```python
from build123d import *

# Parameters (mm, degrees)
SKETCH1_W           = 78.74
SKETCH1_H           = 127
SKETCH1_W_2         = 38.1
SKETCH1_H_2         = 44.45
BOSS_EXTRUDE1_DEPTH = 2.54
BOSS_EXTRUDE2_DEPTH = 44.45
CUT_EXTRUDE1_REACH  = 129
SKETCH3_W           = 9.5
SKETCH3_H           = 11.5
SKETCH3_W_2         = 13
CUT_EXTRUDE2_REACH  = 103.6
CUT_EXTRUDE3_REACH  = 121.38
SKETCH6_R           = 3
SKETCH29_R          = 9.144
SKETCH29_R_2        = 6.604
CUT_EXTRUDE8_DEPTH  = 2.54


with BuildPart() as part:
    # Sketch1 → Boss-Extrude1 (new body)
    with BuildSketch(Plane(origin=(0, 0, 0), x_dir=(1, 0, 0), z_dir=(0, 1, 0))):
        with Locations((39.37, 63.5)):
            Rectangle(SKETCH1_W, SKETCH1_H)
        with Locations((97.79, 104.775)):
            Rectangle(SKETCH1_W_2, SKETCH1_H_2)
        Polygon((116.84, 127), (116.84, 82.55), (116.84, 0), (177.8, 0), (177.8, 127), align=None)
    extrude(amount=BOSS_EXTRUDE1_DEPTH)

    # Sketch2 → Boss-Extrude2 (add)
    with BuildSketch(Plane(origin=(0, 2.54, 0), x_dir=(1, 0, 0), z_dir=(0, 1, 0))):
        Polygon((0, 127), (0, 0), (78.74, 0), (78.74, 82.55), (116.84, 82.55), (116.84, 0), (177.8, 0), (177.8, 127), align=None)
        Polygon((119.38, 2.54), (175.26, 2.54), (175.26, 124.46), (2.54, 124.46), (2.54, 2.54), (76.2, 2.54), (76.2, 85.09), (119.38, 85.09), align=None, mode=Mode.SUBTRACT)
    extrude(amount=BOSS_EXTRUDE2_DEPTH)

    # Sketch3 → Cut-Extrude1 (cut, up to next)
    with BuildSketch(Plane(origin=(0, 0, -127), x_dir=(-1, 0, 0), z_dir=(0, 0, -1)), mode=Mode.PRIVATE) as cut_extrude1_sk1:
        with Locations((-13.64, 16.24)):
            Rectangle(SKETCH3_W, SKETCH3_H)
    cut_extrude1_tool1 = extrude(cut_extrude1_sk1.sketch, amount=-CUT_EXTRUDE1_REACH, mode=Mode.PRIVATE) & part.part
    add(cut_extrude1_tool1.solids().sort_by_distance((13.64, 16.24, -127))[0], mode=Mode.SUBTRACT)
    # Sketch3 → Cut-Extrude1 (cut, up to next)
    with BuildSketch(Plane(origin=(0, 0, -127), x_dir=(-1, 0, 0), z_dir=(0, 0, -1)), mode=Mode.PRIVATE) as cut_extrude1_sk2:
        with Locations((-42.39, 16.24)):
            Rectangle(SKETCH3_W_2, SKETCH3_H)
    cut_extrude1_tool2 = extrude(cut_extrude1_sk2.sketch, amount=-CUT_EXTRUDE1_REACH, mode=Mode.PRIVATE) & part.part
    add(cut_extrude1_tool2.solids().sort_by_distance((42.39, 16.24, -127))[0], mode=Mode.SUBTRACT)

    # Sketch5 → Cut-Extrude2 (cut, up to next)
    with BuildSketch(Plane.ZY.offset(-76.2), mode=Mode.PRIVATE) as cut_extrude2_sk1:
        with BuildLine():
            Line((-44.315, 27.265), (-43.315, 27.265))
            ThreePointArc((-43.315, 27.265), (-40.815, 24.765), (-43.315, 22.265))
            Line((-43.315, 22.265), (-44.315, 22.265))
            ThreePointArc((-44.315, 22.265), (-46.815, 24.765), (-44.315, 27.265))
        make_face()
    cut_extrude2_tool1 = extrude(cut_extrude2_sk1.sketch, amount=-CUT_EXTRUDE2_REACH, mode=Mode.PRIVATE) & part.part
    add(cut_extrude2_tool1.solids().sort_by_distance((76.2, 24.765, -43.815))[0], mode=Mode.SUBTRACT)

    # Sketch6 → Cut-Extrude3 (cut, up to next)
    with BuildSketch(Plane(origin=(119.38, 0, 0), x_dir=(0, 0, -1), z_dir=(1, 0, 0)), mode=Mode.PRIVATE) as cut_extrude3_sk1:
        with Locations((43.815, 24.765)):
            Circle(SKETCH6_R)
    cut_extrude3_tool1 = extrude(cut_extrude3_sk1.sketch, amount=-CUT_EXTRUDE3_REACH, mode=Mode.PRIVATE) & part.part
    add(cut_extrude3_tool1.solids().sort_by_distance((119.38, 24.765, -43.815))[0], mode=Mode.SUBTRACT)

    # Sketch29 → Cut-Extrude8 (cut)
    with BuildSketch(Plane.XY):
        with Locations((57.15, 23.495)):
            Circle(SKETCH29_R)
        with Locations((19.05, 23.495)):
            Circle(SKETCH29_R_2)
    extrude(amount=-CUT_EXTRUDE8_DEPTH, mode=Mode.SUBTRACT)


solid = part.part
```
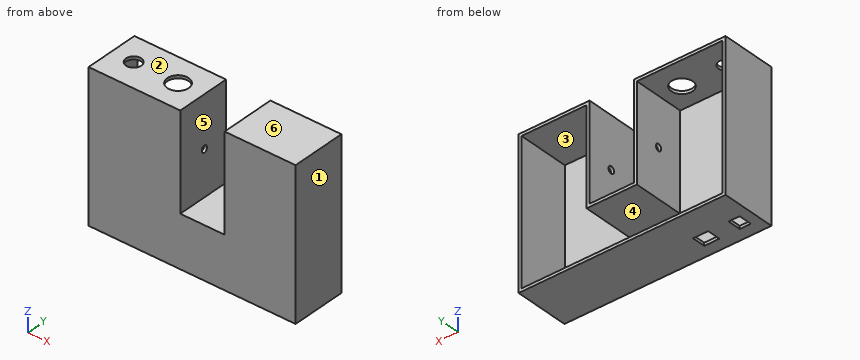
Build history of the part. All positions in model axes, mm. Face numbers are marked on the shaded views. A direction names the side the tool comes from. Give positions to 0.01 mm unless a question says otherwise; leave off trailing zeros. Loops run counter-clockwise (first coordinate to the right, second up) from the corner with the lowest first, then second, coordinate; pieces in that order, holes last.
1) Probe line 1 along X through (y, z) = (10, -41); line 2 along X through (y, z) = (13, -106); line 3 along Z through (x, y) = (126, 29). List the from-to ranges inside material, lowest first.
Values follow:
line 1: x = 0 to 2.54, 76.2 to 78.74, 116.84 to 119.38, 175.26 to 177.8
line 2: x = 0 to 2.54, 175.26 to 177.8
line 3: z = -127 to -124.46, -2.54 to 0
2) Drop flat-ended pins along their axis: P1, Ø1.5, axis at x = 74, z = -15, coming from the +Y side; P2, Ø12, axis at x = 93, y = 20, coming from the +Z side. Give the stop position or say it passes through.
Values follow:
P1: stops at y = 2.54
P2: stops at z = -82.55
3) Band-saw the part on D-D on x = 114.5. List the corners of the cut face in (y, z).
Values follow:
outline: (0, -127) - (46.99, -127) - (46.99, -124.46) - (2.54, -124.46) - (2.54, -85.09) - (46.99, -85.09) - (46.99, -82.55) - (0, -82.55) - close
4) 3-axis set-ups, long thin cutter, end or side, ignore diameter. For the marked faces 4, 5 and 6: which of +Z, -Z, +X, -X, +Y, -Y reach the whole face in a straight line?
Values follow:
face 4: +Y
face 5: +Z, +Y, -Y
face 6: +Z, +X, -X, +Y, -Y
5) Band-saw the part on C-C on z = -65.5. List the corners of the cut face in (x, y).
Values follow:
outline: (0, 0) - (78.74, 0) - (78.74, 46.99) - (76.2, 46.99) - (76.2, 2.54) - (2.54, 2.54) - (2.54, 46.99) - (0, 46.99) - close; (116.84, 0) - (177.8, 0) - (177.8, 46.99) - (175.26, 46.99) - (175.26, 2.54) - (119.38, 2.54) - (119.38, 46.99) - (116.84, 46.99) - close
6) Band-saw the part on A-A on y = 34.5. List the corners of the cut face in (x, z), then the cut area to 3 significant figures.
Values follow:
outline: (0, -127) - (177.8, -127) - (177.8, 0) - (116.84, 0) - (116.84, -82.55) - (78.74, -82.55) - (78.74, 0) - (0, 0) - close; hole (2.54, -124.46) - (175.26, -124.46) - (175.26, -2.54) - (119.38, -2.54) - (119.38, -85.09) - (76.2, -85.09) - (76.2, -2.54) - (2.54, -2.54) - close
area: 1,940 mm2
7) Two-plate mould, pull along X, no slides. Class the marked faces 1, 2 and 3: released by +X, released by -X, zero draft, split by the parting line, or undercut.
Values follow:
face 1: released by +X
face 2: zero draft
face 3: undercut
8) Band-saw the part on B-B on x = 57.15. List the corners of the cut face in (y, z), then the cut area to 3 significant figures.
Values follow:
outline: (0, -127) - (46.99, -127) - (46.99, -124.46) - (2.54, -124.46) - (2.54, -2.54) - (14.35, -2.54) - (14.35, 0) - (0, 0) - close; (32.64, -2.54) - (46.99, -2.54) - (46.99, 0) - (32.64, 0) - close
area: 502 mm2
